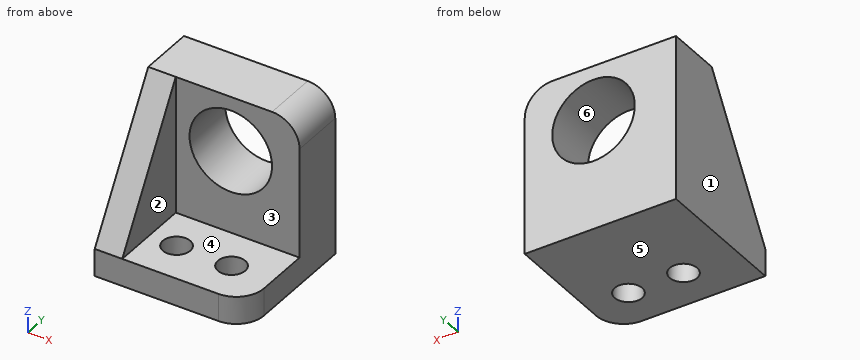
from build123d import *

# Parameters (mm, degrees)
F0_R     = 50
F0_W     = 100
F0_H     = 300
F1_DEPTH = 100
F2_DEPTH = 600
F3_R     = 100
F5_DEPTH = 100
F6_R     = 150
F7_DEPTH = 200


with BuildPart() as f1:
    # F0 (on Top) → F1 (new body)
    with BuildSketch(Plane.XY):
        with BuildLine():
            Line((-175, -250), (175, -250))
            ThreePointArc((175, -250), (245.7106781187, -220.7106781187), (275, -150))
            Line((275, -150), (275, 50))
            Line((275, 50), (-175, 50))
            Line((-175, 50), (-175, -250))
        make_face()
        with Locations((-75, -100)):
            Circle(F0_R, mode=Mode.SUBTRACT)
        with Locations((125, -100)):
            Circle(F0_R, mode=Mode.SUBTRACT)
        Polygon((-275, 50), (-175, 50), (275, 50), (275, 250), (-275, 250), align=None)
        with Locations((-225, -100)):
            Rectangle(F0_W, F0_H)
    extrude(amount=F1_DEPTH)

    # F0 (on Top) → F2 (join)
    with BuildSketch(Plane.XY):
        Polygon((-275, 50), (-175, 50), (275, 50), (275, 250), (-275, 250), align=None)
        with Locations((-225, -100)):
            Rectangle(F0_W, F0_H)
    extrude(amount=F2_DEPTH)

    # F3
    f3_edges = [f1.edges().sort_by_distance(p)[0] for p in [
        (275, 150, 600),
    ]]
    fillet(f3_edges, radius=F3_R)

    # F4 (on face) → F5 (cut)
    with BuildSketch(Plane.YZ.offset(-175)):
        Polygon((-250, 100), (50, 600), (-250, 600), align=None)
    extrude(amount=-F5_DEPTH, mode=Mode.SUBTRACT)

    # F6 (on face) → F7 (cut)
    with BuildSketch(Plane.XZ.offset(-50)):
        with Locations((25, 400)):
            Circle(F6_R)
    extrude(amount=-F7_DEPTH, mode=Mode.SUBTRACT)


solid = f1.part
Build history of the part. All positions in model axes, mm. Face numbers are marked on the shaded views. A direction names the side the tool comes from. Round coordinates to 2 decimals unless told otherwise and drop trailing zeros. Loops run counter-clockwise (first coordinate to the right, second up) from the corner with the lowest first, then second, coordinate; pieces in that order, holes last. Notation, with made-up numbers: (31, -19.75) -> (74, -19.75) arc R26 cw to (74, 16.25) -> close; hole circle Ø11 at (-7.75, 6.25). An arc over 180 degrees is marked (long way). Answer in a Markdown table with one row per item.
Item 1: Saw through at C-C (x = 25). Write the cut outline in (y, z).
Answers below:
| item | result |
|---|---|
| outline | (-250, 0) -> (250, 0) -> (250, 250) -> (50, 250) -> (50, 100) -> (-250, 100) -> close; (50, 550) -> (250, 550) -> (250, 600) -> (50, 600) -> close |
Item 2: Which spindle directions (+Z, -Z, +X, -X, +Y, -Y) get a long thin tool onto all of the face, cutting with end or side? Do the marked faces 1 and 2. Say none if no direction does.
Answers below:
| item | result |
|---|---|
| face 1 | +Z, -Z, -X, +Y, -Y |
| face 2 | +Z, +X, -Y |
Item 3: Saw through at A-A (y = -100). Write the cut outline in (x, z), and give its area (3 significant figures).
Answers below:
| item | result |
|---|---|
| outline | (-275, 0) -> (-125, 0) -> (-125, 100) -> (-175, 100) -> (-175, 350) -> (-275, 350) -> close; (-25, 0) -> (75, 0) -> (75, 100) -> (-25, 100) -> close; (175, 0) -> (275, 0) -> (275, 100) -> (175, 100) -> close |
| area | 60,000 mm² |
Item 4: Saw through at D-D (y = 111.5). Write the cut outline in (x, z).
Answers below:
| item | result |
|---|---|
| outline | (-275, 0) -> (275, 0) -> (275, 500) arc R100 ccw to (175, 600) -> (-275, 600) -> close; hole circle Ø300 at (25, 400) |
Item 5: Saw through at B-B (z = 400). Write the cut outline in (x, y).
Answers below:
| item | result |
|---|---|
| outline | (-275, -70) -> (-175, -70) -> (-175, 50) -> (-125, 50) -> (-125, 250) -> (-275, 250) -> close; (175, 50) -> (275, 50) -> (275, 250) -> (175, 250) -> close |
Item 6: Drill centre lines: L1, parallel to Y at x = 125, z = 68; L2, parallel to Z at x = 25, y = 202.5; L3, parallel to Y at x = -3.5, z = 201. Where is each one in solid material? Low to high. Write a range as [from, to].
Answers below:
| item | result |
|---|---|
| L1 | y = [-250, -150], [-50, 250] |
| L2 | z = [0, 250], [550, 600] |
| L3 | y = [50, 250] |
Item 7: Pin check, flat tips, straight feed: pin 1 (5 mm diameter, centred on x = -193, z = 519.5, fed in from -Y); pin 2 (1 mm diameter, centred on y = 45.5, z = 524.5, fed in from +X); pin 3 (8 mm diameter, centred on x = 111.5, y = 101.5, fed in from -Z); pin 4 (12 mm diameter, centred on x = 183.5, z = 465.5, fed in from -Y). Stop position of each tip, or through.
Answers below:
| item | result |
|---|---|
| pin 1 | stops at y = 0.2 |
| pin 2 | stops at x = -175 |
| pin 3 | stops at z = 0 |
| pin 4 | stops at y = 50 |
Item 8: Mould opens along Z. For the marked faces 3, 4, 5 and 6 say: +Z half, -Z half, draft (parallel to the pull), parting line (faces both ways), or undercut.
Answers below:
| item | result |
|---|---|
| face 3 | draft |
| face 4 | +Z half |
| face 5 | -Z half |
| face 6 | undercut |
